Autodesk Inventor part; units mm, degrees
ref_plane "YZ Plane" through (0, 0, 0) normal (1, 0, 0) x (0, 1, 0)
ref_plane "XZ Plane" through (0, 0, 0) normal (0, 1, 0) x (-1, 0, 0)
ref_plane "XY Plane" through (0, 0, 0) normal (0, 0, 1) x (1, 0, 0)
sketch "Эскиз1" plane through (0, 0, 0) normal (0, 0, 1) x (1, 0, 0)
  line L0 (0, 0) -> (-20, 0) construction
  line L1 (-20, 0) -> (-20, 10) construction
  line L2 (-20, 10) -> (0, 10) construction
  line L3 (0, 10) -> (0, 0) construction
  line L4 (-20, 0) -> (8.2, 0) construction
  line L5 (8.2, 0) -> (8.2, 16)
  line L6 (8.2, 16) -> (-20, 16)
  line L7 (-20, 16) -> (-20, 0) construction
  line L8 (-20, 16) -> (-20, 10)
  line L9 (-20, 10) -> (0, 10)
  line L10 (0, 10) -> (0, 0)
  line L11 (0, 0) -> (8.2, 0)
  point P0 (-10, 10)
  dimension "d0" = 20
  dimension "d1" = 10
  dimension "d2" = 6
  dimension "d3" = 8.2
extrude "Выдавливание1" add sketch "Эскиз1" along normal blind 56
sketch "Эскиз5" plane through (-20, 10, 0) normal (-1, 0, 0) x (0, 0, 1)
  line L0 (0, 0) -> (56, 0)
  line L1 (0, -10) -> (56, -10)
  line L2 (56, 0) -> (48, 0)
  line L3 (48, 0) -> (48, -10)
  line L4 (48, -10) -> (56, -10)
  line L5 (56, -10) -> (56, 0)
  line L6 (0, 0) -> (8, 0)
  line L7 (8, 0) -> (8, -10)
  line L8 (8, -10) -> (0, -10)
  line L9 (0, -10) -> (0, 0)
  point P0 (48, 0)
  point P1 (8, -10)
  point P2 (8, 0)
  dimension "d37" = 8
  dimension "d38" = 8
extrude "Выдавливание5" add sketch "Эскиз5" against normal blind 5.2 contours L0 L7 L1 L9 | L0 L5 L1 L3
sketch "Эскиз6" plane through (-20, 0, 48) normal (0, -1, 0) x (1, 0, 0)
  line L0 (0, 0) -> (0, 8)
  line L1 (0, 0) -> (5.2, 0)
  line L2 (5.2, 8) -> (5.2, 0)
  line L3 (0, 8) -> (5.2, 8)
  circle A0 centre (2.6, 2) radius 1.6
  line L4 (2.6, 2) -> (5.2, 4)
  line L5 (2.6, 2) -> (0, 4)
  line L6 (0, 0) -> (0, 8)
  point P0 (20, -48)
  dimension "d41" = 3.2
  dimension "d45" = 6
extrude "Выдавливание6" cut sketch "Эскиз6" against normal blind 20 contours L5 L4 A0 | A0 L4 L5
sketch "Эскиз7" plane through (-20, 16, 0) normal (0, 1, 0) x (1, 0, 0)
  circle A0 centre (2.6, -50) radius 1.6
  line L0 (5.35, -48.4123) -> (5.35, -51.5877)
  line L1 (5.35, -51.5877) -> (2.6, -53.1754)
  line L2 (2.6, -53.1754) -> (-0.15, -51.5877)
  line L3 (-0.15, -51.5877) -> (-0.15, -48.4123)
  line L4 (-0.15, -48.4123) -> (2.6, -46.8246)
  line L5 (2.6, -46.8246) -> (5.35, -48.4123)
  line L6 (0, 0) -> (0, -56)
  point P0 (20, 0)
  point P1 (0, -48.3257)
  point P2 (0, -51.6743)
  dimension "d44" = 5.5
extrude "Выдавливание7" cut sketch "Эскиз7" against normal blind 2.4 contours L0 L1 L2 L6 L4 L5
ref_plane "РабПлоскость1" through (0, 0, 28) normal (0, 0, 1) x (1, 0, 0)
mirror "Зеркальное отражение1" about plane through (0, 0, 28) normal (0, 0, 1) of "Выдавливание6", "Выдавливание7"
sketch "Эскиз8" plane through (-20, 16, 0) normal (0, 1, 0) x (1, 0, 0)
  circle A0 centre (24.8, -52) radius 1.6
  circle A1 centre (24.8, -18) radius 1.6 construction
  line L0 (24.8, -52) -> (24.8, -18)
  line L1 (28.2, 0) -> (28.2, -56)
  line L2 (0, -7.6743) -> (0, -48.3257)
  line L3 (28.2, -56) -> (0, -56)
  point P0 (20, 0)
  dimension "d49" = 3.2
  dimension "d50" = 3.2
  dimension "d51" = 34
  dimension "d52" = 24.8
  dimension "d53" = 4
extrude "Выдавливание8" cut sketch "Эскиз8" against normal blind 56
sketch "Эскиз9" plane through (-20, 16, 0) normal (0, 1, 0) x (1, 0, 0)
  circle A0 centre (9.8, 137.0813) radius 6
  line L0 (15.8, 137.0813) -> (15.8, -29.0562) construction
  circle A1 centre (21.8, -18) radius 6 construction
  circle A2 centre (21.8, -18) radius 2.1
  point P0 (20, 0)
  dimension "d56" = 12
  dimension "d57" = 18
  dimension "d58" = 4.2
extrude "Выдавливание9" cut sketch "Эскиз9" against normal blind 5 contours A2
equation "\"Радиус_гибки\" = Толщина"
equation "\"Ширина_просечки\" = Толщина"
equation "\"Глубина_просечки\" = 0.5 * Толщина"
equation "\"Размер_просечки\" = 4 * Толщина"
equation "\"Мин_остаток\" = 2 * Толщина"
equation "\"Радиус_перехода\" = Радиус_гибки"
equation "\"Радиус_Якоби\" = Радиус_гибки"
equation "\"Размер_зазора\" = Толщина"
properties part number "креп_центр_м2" material "Полипропилен"
For this review, take the finished solid that the model builds, in its own axes (mm). A direction names the side the tool comes from. Round coordinates to 2 decimals unless told otherwise and drop trailing zeros. Order: outer loops, then holes, each group sorted by start corner. A loop starts at its lowest first (then second) coordinate and runs counter-clockwise, first axis right, second up. Notation, with made-up numbers: M 5.25,28 L 54.25,28 A23 ccw 54.25,50 Z; hole C 21,83 d4. An arc over 180 degrees is marked long. Use a Markdown table: item, result. Add a question column.
Item 1: Add section D-D, the plane y = 12.75. Give the boundary of the cut face in (x, z), then the cut area to 3 significant figures.
Item 2: Tool access review of faces 4 (the flat face through (-18.718, 14.817, 3.586)), 5 (the flat face through (-17, 5, 8)), 6 (the flat face through (-14.8, 5, 52)), 7 (the flat face through (-14.65, 15, 50)), 8 (the flat face through (-6, 12, 0)): name each direction out of +Z, -Z, +X, -X, +Y, -Y from which nothing blocks a thin tool from reaching the whole face with its end or side.
Item 3: Mouldability with a two-part tool opening along Z and no side actions: class faces 1 (the cylindrical face through (-17.75, 6.7, 4.44)), 2 (the flat face through (-6, 12, 56)), 3 (the flat face through (-17, 0, 52)) as released by +Z, released by -Z, zero draft, split by the parting line, or undercut.
Item 4: Add section C-C, the plane z = 18. Give the boundary of the cut face in (x, y).
Item 5: Add section A-A, the plane y = 3.5. Give the boundary of the cut face in (x, z), then the cut area to 3 significant figures.
Item 6: Add section B-B, the plane x = 4.8. Give the boundary of the cut face in (y, z).
Item 7: To check wall thickness, follow line 1 along X through (y, z) = (4.25, 52); line 2 along Z through (x, y) = (5, 5); line 3 along Z through (x, y) = (-17.4, 8.5). State the ranges of each line that lie inside material, in increasing order.
Item 8: Insertion check: pin 1 (4 mm diameter, centred on x = -12.5, z = 36.5, fed in from -Y); pin 2 (4.5 mm diameter, centred on x = -17.5, z = 50, fed in from +Y); pin 3 (2.5 mm diameter, centred on x = 1.8, z = 18, fed in from +Y). Each pin has a flat end and moves straight along its axis. Give the tip position at first contact, or say it passes through.
Geometry results:
| question | item | result |
|---|---|---|
| 1 | outline | M -20,0 L 8.2,0 L 8.2,56 L -20,56 Z; hole C -17.4,6 d3.2; hole C -17.4,50 d3.2; hole C 1.8,18 d4.2; hole C 4.8,52 d3.2 |
| 1 | area | 1,540 mm² |
| 2 | face 4 | +Y |
| 2 | face 5 | -X, -Y |
| 2 | face 6 | +Z, -Z, -Y |
| 2 | face 7 | -X, +Y |
| 2 | face 8 | -Z, +X, -X, +Y, -Y |
| 3 | face 1 | undercut |
| 3 | face 2 | released by +Z |
| 3 | face 3 | zero draft |
| 4 | outline | M -20,10 L 0,10 L 0,0 L 8.2,0 L 8.2,16 L 3.9,16 L 3.9,11 L -0.3,11 L -0.3,16 L -20,16 Z |
| 5 | outline | M -20,0 L -14.8,0 L -14.8,8 L -20,8 Z; M -20,48 L -14.8,48 L -14.8,56 L -20,56 Z; M 0,0 L 8.2,0 L 8.2,56 L 0,56 Z; hole C -17.4,6 d3.2; hole C -17.4,50 d3.2; hole C 4.8,52 d3.2 |
| 5 | area | 518 mm² |
| 6 | outline | M 0,0 L 16,0 L 16,50.4 L 0,50.4 Z; M 0,53.6 L 16,53.6 L 16,56 L 0,56 Z |
| 7 | line 1 | x = -20 to -14.8, 0 to 3.2, 6.4 to 8.2 |
| 7 | line 2 | z = 0 to 50.41, 53.59 to 56 |
| 7 | line 3 | z = 0 to 4.4, 7.6 to 8, 48 to 48.4, 51.6 to 56 |
| 8 | pin 1 | stops at y = 10 |
| 8 | pin 2 | stops at y = 13.6 |
| 8 | pin 3 | stops at y = 11 |
